Autodesk Fusion 360 part; units mm, degrees
sketch "Sketch2" plane through (0, 0, 0) normal (0, 0, 1) x (1, 0, 0) in component "jig"
  line L0 (0, 0) -> (0, 66.75)
  line L1 (0, 66.75) -> (146.025, 66.75)
  line L2 (146.025, 66.75) -> (146.025, 0)
  line L3 (146.025, 0) -> (0, 0)
  line L4 (22.25, 0) -> (41.25, 0)
  line L5 (41.25, 0) -> (41.25, 44.5)
  line L6 (41.25, 44.5) -> (22.25, 44.5)
  line L7 (22.25, 44.5) -> (22.25, 0)
  line L8 (0, 0) -> (22.25, 0)
  line L9 (22.25, 0) -> (22.25, -9.5)
  line L10 (22.25, -9.5) -> (0, -9.5)
  line L11 (0, -9.5) -> (0, 0)
  line L12 (146.025, 0) -> (41.25, 0)
  line L13 (41.25, 0) -> (41.25, -9.5)
  line L14 (41.25, -9.5) -> (146.025, -9.5)
  line L15 (146.025, -9.5) -> (146.025, 0)
  line L16 (22.25, 44.5) -> (0, 44.5) construction
  line L17 (41.25, 44.5) -> (146.025, 44.5) construction
  dimension "d27" = 104.775
  dimension "d29" = 9.5
  dimension "d58" = 19
  dimension "d59" = 22.25
  dimension "d60" = 44.5
  dimension "d64" = 22.25
extrude "Extrude1" add sketch "Sketch2" along normal blind 10 contours L0 L1 L2 L3 L5 L6 L7 L8 L12 in component "jig"
extrude "Extrude2" add sketch "Sketch2" along normal blind 33.75 contours L3 L8 L9 L10 L11 | L3 L12 L13 L14 L15 in component "jig"
sketch "Sketch3" plane through (0, 0, 0) normal (-1, 0, 0) x (0, -1, 0) in component "jig"
  line L0 (-66.75, 0) -> (9.5, 0)
  line L1 (9.5, 0) -> (9.5, 33.75)
  line L2 (9.5, 33.75) -> (0, 33.75)
  line L3 (-160, 13) -> (-160.4879, 12.5121)
  line L4 (-160.2757, 12) -> (-160, 12)
  line L5 (-160, 13) -> (-160, 12)
  arc A0 (-160.4879, 12.5121) -> (-160.2757, 12) centre (-160.2757, 12.3) ccw
  line L6 (0, 10) -> (0.2757, 10)
  line L7 (0.4879, 10.5121) -> (0, 11)
  line L8 (0, 10) -> (0, 11)
  arc A1 (0.2757, 10) -> (0.4879, 10.5121) centre (0.2757, 10.3) ccw
  line L9 (-66.75, 10) -> (-66.75, 0)
  line L10 (0, 33.75) -> (0, 10)
  line L11 (0, 10) -> (-66.75, 10)
  dimension "d34" = 1
  dimension "d35" = 0.3
  dimension "d36" = 45
  dimension "d37" = 1
  dimension "d38" = 45
  dimension "d39" = 0.3
extrude "Extrude3" cut sketch "Sketch3" against normal up to surface (146.025 mm away) contours L6 L7 L8 A1 L10 | L3 L4 L5 A0 in component "jig"
fillet "Fillet2" radius 3.175 2 edges at (22.25, 44.5, 5) (41.25, 44.5, 5) in component "jig"
sketch "Sketch2 (2)" plane through (0, -9.5, 0) normal (0, -1, 0) x (1, 0, 0) in component "jig"
  line L0 (0, 0) -> (22.25, 0)
  line L1 (22.25, 0) -> (22.25, 33.75)
  line L2 (22.25, 33.75) -> (0, 33.75)
  line L3 (0, 33.75) -> (0, 0)
  line L4 (22.25, 33.75) -> (41.25, 33.75)
  line L5 (41.25, 0) -> (41.25, 33.75)
  line L6 (41.25, 33.75) -> (41.25, 29.75)
  line L7 (22.25, 33.75) -> (22.25, 29.75)
  line L8 (22.25, 29.75) -> (24.6335, 31.75)
  line L9 (24.6335, 31.75) -> (38.8665, 31.75)
  line L10 (38.8665, 31.75) -> (41.25, 29.75)
  line L11 (22.25, 29.75) -> (41.25, 29.75) construction
  point P0 (41.25, 33.75)
  dimension "d65" = 50
  dimension "d66" = 50
  dimension "d67" = 4
  dimension "d68" = 2
extrude "Extrude5" add sketch "Sketch2 (2)" against normal up to surface (9.5 mm away) contours L1 L4 L5 L6 L7 L8 L9 L10 in component "jig"
sketch "Sketch3 (2)" plane through (0, 0, 10) normal (0, 0, 1) x (-1, 0, 0) in component "jig"
  line L0 (-25.425, -44.5) -> (-38.075, -44.5)
  arc A0 (-41.25, -41.325) -> (-38.075, -44.5) centre (-38.075, -41.325) ccw
  line L1 (-41.25, -41.325) -> (-41.25, 0.2757)
  line L2 (-41.25, 0.2757) -> (-146.025, 0.2757)
  line L3 (-146.025, 0.2757) -> (-146.025, -66.75)
  line L4 (-146.025, -66.75) -> (0, -66.75)
  line L5 (0, -66.75) -> (0, 0.2757)
  line L6 (0, 0.2757) -> (-22.25, 0.2757)
  line L7 (-22.25, 0.2757) -> (-22.25, -41.325)
  arc A1 (-25.425, -44.5) -> (-22.25, -41.325) centre (-25.425, -41.325) ccw
  line L8 (-56.25, -56.75) -> (-131.025, -56.75)
  line L9 (-136.025, -51.75) -> (-136.025, -38.625)
  line L10 (-131.025, -33.625) -> (-56.25, -33.625)
  line L11 (-51.25, -38.625) -> (-51.25, -51.75)
  line L12 (-146.025, 0) -> (0, 0)
  arc A2 (-56.25, -56.75) -> (-51.25, -51.75) centre (-56.25, -51.75) ccw
  arc A3 (-136.025, -51.75) -> (-131.025, -56.75) centre (-131.025, -51.75) ccw
  arc A4 (-131.025, -33.625) -> (-136.025, -38.625) centre (-131.025, -38.625) ccw
  arc A5 (-51.25, -38.625) -> (-56.25, -33.625) centre (-56.25, -38.625) ccw
  line L13 (-56.25, -0.5) -> (-131.025, -0.5)
  line L14 (-136.025, -5.5) -> (-136.025, -18.625)
  line L15 (-131.025, -23.625) -> (-56.25, -23.625)
  line L16 (-51.25, -18.625) -> (-51.25, -5.5)
  line L17 (0, 9.5) -> (-146.025, 9.5)
  line L18 (-93.6375, -56.75) -> (-93.6375, -33.625) construction
  line L19 (-93.6375, -23.625) -> (-93.6375, -0.5) construction
  arc A6 (-56.25, -23.625) -> (-51.25, -18.625) centre (-56.25, -18.625) ccw
  arc A7 (-51.25, -5.5) -> (-56.25, -0.5) centre (-56.25, -5.5) ccw
  arc A8 (-131.025, -0.5) -> (-136.025, -5.5) centre (-131.025, -5.5) ccw
  arc A9 (-136.025, -18.625) -> (-131.025, -23.625) centre (-131.025, -18.625) ccw
  dimension "d71" = 10
  dimension "d72" = 10
  dimension "d74" = 10
  dimension "d75" = 5
  dimension "d89" = 10
  dimension "d90" = 10
  dimension "d91" = 5
extrude "Extrude6" cut sketch "Sketch3 (2)" against normal up to surface (10 mm away) contours L8 L9 L10 L11 A2 A3 A4 A5 | L13 L14 L15 L16 A6 A7 A8 A9 in component "jig"
sketch "Sketch10" plane through (0, 0, 0) normal (0, 1, 0) x (-1, 0, 0) in component "jig"
  line L0 (-146.025, 11) -> (-41.25, 11)
  line L1 (-41.25, 11) -> (-41.25, 29.75)
  line L2 (-41.25, 29.75) -> (-38.8665, 31.75)
  line L3 (-38.8665, 31.75) -> (-24.6335, 31.75)
  line L4 (-24.6335, 31.75) -> (-22.25, 29.75)
  line L5 (-22.25, 29.75) -> (-22.25, 11)
  line L6 (-22.25, 11) -> (0, 11)
  line L7 (0, 11) -> (0, 33.75)
  line L8 (0, 33.75) -> (-146.025, 33.75)
  line L9 (-146.025, 33.75) -> (-146.025, 11)
  line L10 (-146.025, 49.75) -> (-53.25, 49.75)
  line L11 (-51.25, 28.75) -> (-51.25, 21.3333)
  line L12 (-56.25, 16.3333) -> (-146.025, 16.3333)
  line L13 (-146.025, 16.3333) -> (-146.025, 49.75)
  line L14 (-146.025, 10) -> (0, 10)
  line L15 (0, 49.75) -> (-10.25, 49.75)
  line L16 (-12.25, 28.75) -> (-12.25, 21.3333)
  line L17 (-7.25, 16.3333) -> (0, 16.3333)
  line L18 (0, 16.3333) -> (0, 49.75)
  line L19 (-53.25, 49.75) -> (-10.25, 49.75)
  line L20 (-17.25, 33.75) -> (-46.25, 33.75)
  arc A0 (-56.25, 16.3333) -> (-51.25, 21.3333) centre (-56.25, 21.3333) ccw
  arc A1 (-46.25, 33.75) -> (-51.25, 28.75) centre (-46.25, 28.75) ccw
  arc A2 (-12.25, 28.75) -> (-17.25, 33.75) centre (-17.25, 28.75) ccw
  arc A3 (-12.25, 21.3333) -> (-7.25, 16.3333) centre (-7.25, 21.3333) ccw
  dimension "d81" = 10
  dimension "d82" = 6.3333
  dimension "d83" = 6.3333
  dimension "d84" = 10
  dimension "d85" = 16
  dimension "d86" = 5
extrude "Extrude7" cut sketch "Sketch10" against normal up to surface (9.5 mm away) contours L8 L9 L11 L12 L13 A0 A1 | L7 L8 L16 L17 L18 A2 A3 in component "jig"
fillet "Fillet3" radius 5 4 edges at (0, -4.75, 16.3333) (0, 66.75, 5) (146.025, -4.75, 16.3333) (146.025, 66.75, 5) in component "jig"
sketch "Sketch11" plane through (0, 0, 10) normal (0, 0, 1) x (-1, 0, 0) in component "jig"
  arc A0 (-146.025, -61.75) -> (-141.025, -66.75) centre (-141.025, -61.75) ccw
  line L0 (-141.025, -66.75) -> (-5, -66.75)
  arc A1 (-5, -66.75) -> (0, -61.75) centre (-5, -61.75) ccw
  line L1 (0, -61.75) -> (0, 0.2757)
  line L2 (0, 0.2757) -> (-22.25, 0.2757)
  line L3 (-22.25, 0.2757) -> (-22.25, -41.325)
  arc A2 (-25.425, -44.5) -> (-22.25, -41.325) centre (-25.425, -41.325) ccw
  line L4 (-25.425, -44.5) -> (-38.075, -44.5)
  arc A3 (-41.25, -41.325) -> (-38.075, -44.5) centre (-38.075, -41.325) ccw
  line L5 (-41.25, -41.325) -> (-41.25, 0.2757)
  line L6 (-41.25, 0.2757) -> (-146.025, 0.2757)
  line L7 (-146.025, 0.2757) -> (-146.025, -61.75)
  line L8 (-136.025, -51.75) -> (-136.025, -38.625)
  arc A4 (-131.025, -33.625) -> (-136.025, -38.625) centre (-131.025, -38.625) ccw
  line L9 (-131.025, -33.625) -> (-56.25, -33.625)
  arc A5 (-51.25, -38.625) -> (-56.25, -33.625) centre (-56.25, -38.625) ccw
  line L10 (-51.25, -38.625) -> (-51.25, -51.75)
  arc A6 (-56.25, -56.75) -> (-51.25, -51.75) centre (-56.25, -51.75) ccw
  line L11 (-56.25, -56.75) -> (-131.025, -56.75)
  arc A7 (-136.025, -51.75) -> (-131.025, -56.75) centre (-131.025, -51.75) ccw
  line L12 (-131.025, -0.5) -> (-56.25, -0.5)
  arc A8 (-51.25, -5.5) -> (-56.25, -0.5) centre (-56.25, -5.5) ccw
  line L13 (-51.25, -5.5) -> (-51.25, -18.625)
  arc A9 (-56.25, -23.625) -> (-51.25, -18.625) centre (-56.25, -18.625) ccw
  line L14 (-56.25, -23.625) -> (-131.025, -23.625)
  arc A10 (-136.025, -18.625) -> (-131.025, -23.625) centre (-131.025, -18.625) ccw
  line L15 (-136.025, -18.625) -> (-136.025, -5.5)
  arc A11 (-131.025, -0.5) -> (-136.025, -5.5) centre (-131.025, -5.5) ccw
  line L16 (0, -10) -> (-12.25, -10)
  line L17 (-12.25, -10) -> (-12.25, -54.5)
  line L18 (-12.25, -54.5) -> (-41.25, -54.5)
  line L19 (-41.25, -54.5) -> (-41.25, -66.75)
  line L20 (0, -10) -> (0, -66.75)
  line L21 (0, -66.75) -> (-41.25, -66.75)
  line L22 (-46.25, 0) -> (-17.25, 0)
  dimension "d94" = 10
  dimension "d95" = 10
  dimension "d96" = 10
extrude "Extrude8" cut sketch "Sketch11" against normal up to surface (10 mm away) contours L0 A1 L1 L16 L17 L18 L19 L20 L21 in component "jig"
fillet "Fillet4" radius 5 5 edges at (41.25, 66.75, 5) (41.25, 54.5, 5) (12.25, 54.5, 5) (12.25, 10, 5) (0, 10, 5) in component "jig"
fillet "Fillet5" radius 2 4 edges at (22.25, -4.75, 29.75) (24.6335, -4.75, 31.75) (38.8665, -4.75, 31.75) (41.25, -4.75, 29.75) in component "jig"
component "jig" placed x (1, 0, 0) y (0, 1, 0) z (0, 0, 1) at (0, 0, 0)
equation "stockW = 200 mm"
equation "stockH = 89 mm"
equation "stockT = 19 mm"
equation "lipT = stockT / 2"
equation "lipH = lipT * 2 / 3"
equation "jigT = 10 mm"
equation "stock2H = 160 mm"
equation "baseMargin = 3.125 in + 1\""
equation "d27 = baseMargin"
equation "d29 = lipT"
equation "d30 = jigT"
equation "d32 = jigT + stockT * 1.25"
equation "d58 = stockT"
equation "d59 = d60 / 2"
equation "d60 = stockH / 2"
equation "jigR = 0.125 in"
equation "d63 = jigR"
equation "d64 = d59"
equation "d66 = d65"
equation "d71 = cutoutOffset"
equation "d72 = d71"
equation "d74 = d71"
equation "d75 = cutoutRadius"
equation "cutoutOffset = 10 mm"
equation "cutoutRadius = 5 mm"
equation "d81 = cutoutOffset"
equation "d82 = lipH"
equation "d83 = lipH"
equation "d84 = cutoutOffset"
equation "d86 = cutoutRadius"
equation "d89 = cutoutOffset"
equation "d90 = cutoutOffset"
equation "d91 = d75"
equation "d93 = cutoutRadius"
equation "d94 = cutoutOffset"
equation "d95 = cutoutOffset"
equation "d96 = cutoutOffset"
equation "d100 = cutoutRadius"
Work out the finished part from the listing and answer in its coordinate system (mm). A direction names the side the tool comes from. Round coordinates to 2 decimals unless told otherwise and drop trailing zeros. Write each loop counter-clockwise with the first axis right and the second up, starting at its lowest first coordinate (ties: lowest second). Pieces come first, ordered by that corner, then holes.
1) Consider probe 1 along Y at (x, z) = (132, 13.5); probe 2 along X at (y, z) = (-6, 4) (3 decimals); probe 3 along X at (y, z) = (3, 4) (3 decimals). Determine where each line is inside the solid, lowest interval first.
2) A cutting plane is placed at C-C on x = 83. Determine the outline of the cut face in (y, z) (3 decimals).
3) A cutting plane is placed at A-A on z = 26. Determine the outline of the cut face in (x, y).
4) Determine the mould class of faces 1 (the face through (52.75, 55.32, 5.07)), 2 (the face through (51.25, 45, 5)), 3 (the face through (52.75, -4.68, 17.76)), 4 (the face through (62, 0, 15)) for opening direction X: pulls with the +X half, pulls with the -X half, needs draft (parallel to the pull), parting line crosses it, or undercut.
5) Which of the six approach directions +Z, -Z, +X, -X, +Y, -Y give full straight-line access (tool end or side, diameter ignored) to faces 5 (the face through (94, 23.625, 5)), 6 (the face through (93, 66.75, 5)), 7 (the face through (23.2, 43.59, 5.07))?
6) A cutting plane is placed at D-D on y = 43. Determine the outline of the cut face in (x, z) (3 decimals), and give its area (3 significant figures).
7) A cutting plane is placed at B-B on y = 30. Determine the outline of the cut face in (x, z) (3 decimals).
8) Flat-ended cylindrical pins translate along their axes: P1, Ø3, axis at x = 114, y = -3, coming from the +Z side; P2, Ø11, axis at y = 26, z = 7, coming from the -X side; P3, Ø5, axis at x = 30, y = -6, coming from the -Z side. Find the tip coordinate at first contact, or state that the pin passes through.
Entries:
1. probe 1: y = -9.5 to 0
1. probe 2: x = 0 to 22.25, 41.25 to 146.025
1. probe 3: x = 0 to 22.25, 41.25 to 51.92, 135.355 to 146.025
2. outline: (-9.5, 0) - (0.5, 0) - (0.5, 10) - (-0.276, 10) arc R0.3 cw to (-0.488, 10.512) - (0, 11) - (0, 16.333) - (-9.5, 16.333) - close; (23.625, 0) - (33.625, 0) - (33.625, 10) - (23.625, 10) - close; (56.75, 0) - (66.75, 0) - (66.75, 10) - (56.75, 10) - close
3. outline: (12.25, -9.5) - (22.25, -9.5) - (22.25, 0) - (12.25, 0) - close; (41.25, -9.5) - (51.25, -9.5) - (51.25, 0) - (41.25, 0) - close
4. face 1: undercut
4. face 2: undercut
4. face 3: pulls with the +X half
4. face 4: needs draft
5. face 5: +Z, -Z
5. face 6: +Z, -Z, +X, -X, +Y
5. face 7: +Z, -Z, -Y
6. outline: (12.25, 0) - (22.728, 0) - (22.728, 10) - (12.25, 10) - close; (40.772, 0) - (51.25, 0) - (51.25, 10) - (40.772, 10) - close; (136.025, 0) - (146.025, 0) - (146.025, 10) - (136.025, 10) - close
6. area: 310 mm2
7. outline: (12.25, 0) - (22.25, 0) - (22.25, 10) - (12.25, 10) - close; (41.25, 0) - (146.025, 0) - (146.025, 10) - (41.25, 10) - close
8. P1: stops at z = 16.33
8. P2: stops at x = 12.25
8. P3: stops at z = 31.75
